Verification items for the finished model (mm, model axes). Face numbers are marked on the shaded views. A direction names the side the tool comes from. Coordinates: 2 decimals unless noted, no trailing zeros. Write each loop counter-clockwise with the first axis right and the second up, starting at its lowest first coordinate (ties: lowest second). Pieces come first, ordered by that corner, then holes. Notation, with made-up numbers: M 77.5,-11 L 88.5,-11 A30 ccw 88.5,19 Z; hole C -31,30.25 d1. An arc over 180 degrees is marked long. Answer in a Markdown table with one row per item.
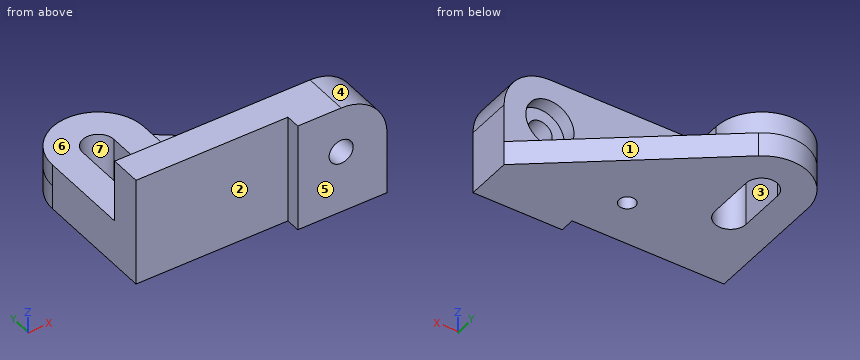
from build123d import *

# Parameters (mm, degrees)
BOSS_EXTRUDE1_DEPTH = 45
BOSS_EXTRUDE2_DEPTH = 10
BOSS_EXTRUDE3_DEPTH = 9
CUT_EXTRUDE1_DEPTH  = 119.004237212
FILLET1_R           = 19
HOLE1_D             = 10
HOLE1_CBORE_D       = 20
HOLE1_CBORE_DEPTH   = 6
M8_TAPPED_HOLE2_D   = 6.8


with BuildPart() as part:
    # Sketch1 → Boss-Extrude1 (new body)
    with BuildSketch(Plane.XY):
        Polygon((0, 0), (0, -13), (63, -13), (63, -19), (100, -19), (100, 0), align=None)
    extrude(amount=BOSS_EXTRUDE1_DEPTH)

    # Sketch2 → Boss-Extrude2 (add)
    with BuildSketch(Plane(origin=(0, 0, 0), x_dir=(-1, 0, 0), z_dir=(0, 0, -1))):
        with BuildLine():
            Line((0, 0), (0, 38))
            ThreePointArc((0, 38), (-10.580703715, 55.032775759), (-30.538468428, 53.095156386))
            Line((-30.538468428, 53.095156386), (-100, 0))
            Line((-100, 0), (0, 0))
        make_face()
    extrude(amount=-BOSS_EXTRUDE2_DEPTH)

    # Sketch4 → Boss-Extrude3 (add)
    with BuildSketch(Plane.XY.offset(10)):
        with BuildLine():
            Line((0, 0), (0, 38))
            ThreePointArc((0, 38), (19, 57), (38, 38))
            Line((38, 38), (38, 0))
            Line((38, 0), (0, 0))
        make_face()
    extrude(amount=BOSS_EXTRUDE3_DEPTH)

    # Sketch5 → Cut-Extrude1 (cut, through all)
    with BuildSketch(Plane.XY.offset(19)):
        with BuildLine():
            Line((25.5, 38), (25.5, 19))
            ThreePointArc((25.5, 19), (19, 12.5), (12.5, 19))
            Line((12.5, 19), (12.5, 38))
            ThreePointArc((12.5, 38), (19, 44.5), (25.5, 38))
        make_face()
    extrude(amount=-CUT_EXTRUDE1_DEPTH, mode=Mode.SUBTRACT)

    # Fillet1
    fillet1_edges = [part.edges().sort_by_distance(p)[0] for p in [
        (100, -9.5, 45),
    ]]
    fillet(fillet1_edges, radius=FILLET1_R)

    # Hole1 (through all)
    with Locations(Plane(origin=(81, 0, 26), x_dir=(1, 0, 0), z_dir=(0, 1, 0))):
        with Locations((0, 0)):
            CounterBoreHole(HOLE1_D / 2, HOLE1_CBORE_D / 2, HOLE1_CBORE_DEPTH)

    # M8 Tapped Hole2 (through all)
    with Locations(Plane(origin=(53, 6, 10), x_dir=(1, 0, 0), z_dir=(0, 0, 1))):
        with Locations((0, 0)):
            Hole(M8_TAPPED_HOLE2_D / 2)


solid = part.part
1) Depth check by flat-ended pin: pin 1 (2 mm diameter, centred on y = 20, z = 7, fed in from +X); pin 2 (1 mm diameter, centred on x = 88.5, z = 30.5, fed in from +Y); pin 3 (2 mm diameter, centred on x = 54.5, z = 11.5, fed in from -Y); pin 4 (8 mm diameter, centred on x = 81, z = 26, fed in from -Y). Enter the tip coordinate at first touch or a pass-through.
Response values:
| item | result |
|---|---|
| pin 1 | stops at x = 75.14 |
| pin 2 | stops at y = -6 |
| pin 3 | stops at y = -13 |
| pin 4 | passes through |
2) Release check for a two-part mould opening along Y. For the marked faces 1, 2, 3 and 4 record: +Y half, -Y half, draft (parallel to the pull), parting line (faces both ways), or undercut.
Response values:
| item | result |
|---|---|
| face 1 | +Y half |
| face 2 | -Y half |
| face 3 | undercut |
| face 4 | draft |
3) Sectioned sample at A-A (x = 19). Record the cut outline in (y, z).
Response values:
| item | result |
|---|---|
| outline | M -13,0 L 12.5,0 L 12.5,19 L 0,19 L 0,45 L -13,45 Z; M 44.5,0 L 57,0 L 57,19 L 44.5,19 Z |
4) Thickness scan on L1, parallel to Z at x = 81, y = -1.85; L2, parallel to Z at x = 81, y = -10.25; L3, parallel to Y at x = 14, z = 41. Record the ranges inside material, lowest first. Write a range as [from, to].
Response values:
| item | result |
|---|---|
| L1 | z = [0, 16], [36, 45] |
| L2 | z = [0, 21], [31, 45] |
| L3 | y = [-13, 0] |
5) Sectioned sample at B-B (y = 16). Record the cut outline in (x, z).
Response values:
| item | result |
|---|---|
| outline | M 0,0 L 13.23,0 L 13.23,19 L 0,19 Z; M 24.77,0 L 79.07,0 L 79.07,10 L 38,10 L 38,19 L 24.77,19 Z |
6) Sectioned sample at C-C (z = 3). Record the cut outline in (x, y).
Response values:
| item | result |
|---|---|
| outline | M 0,-13 L 63,-13 L 63,-19 L 100,-19 L 100,0 L 30.54,53.1 A19 ccw 0,38 Z; hole M 12.5,19 A6.5 ccw 25.5,19 L 25.5,38 A6.5 ccw 12.5,38 Z; hole C 53,6 d6.8 |
7) Tool access check on the marked faces 5, 6 and 7. Record the directions out of +Z, -Z, +X, -X, +Y, -Y that give a thin tool (end or side, any length) a straight path to the whole face; none if there is none.
Response values:
| item | result |
|---|---|
| face 5 | +Z, -Z, +X, -X, -Y |
| face 6 | +Z, +X, -X, +Y |
| face 7 | +Z, -Z |
8) Sectioned sample at D-D (z = 23.5). Record the cut outline in (x, y), then the cut area to 3 significant figures.
Response values:
| item | result |
|---|---|
| outline | M 0,-13 L 63,-13 L 63,-19 L 76.67,-19 L 76.67,-6 L 71.32,-6 L 71.32,0 L 0,0 Z; M 85.33,-19 L 100,-19 L 100,0 L 90.68,0 L 90.68,-6 L 85.33,-6 Z |
| area | 1,290 mm² |
